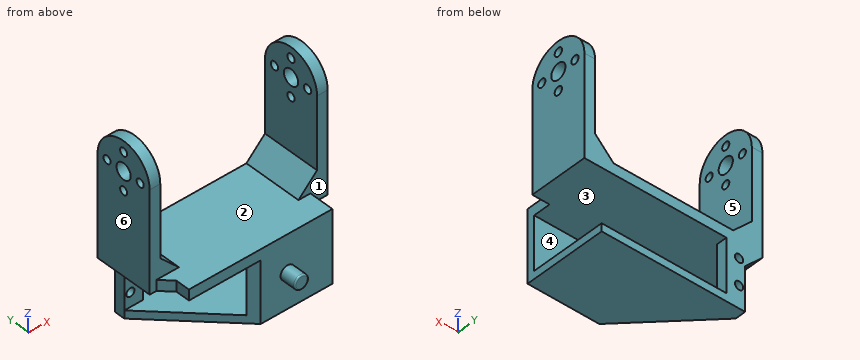
from build123d import *

# Parameters (mm, degrees)
BOSS_EXTRUDE1_DEPTH      = 22
SKETCH3_R                = 1.55
CUT_EXTRUDE1_DEPTH       = 30
CUT_EXTRUDE5_DEPTH       = 9
SKETCH11_R               = 1.55
CUT_EXTRUDE10_DEPTH      = 13
CUT_EXTRUDE11_START      = -10
CUT_EXTRUDE11_DEPTH      = 10
SKETCH13_R               = 3
SKETCH13_R_2             = 1.5
CUT_EXTRUDE12_DEPTH      = 85
FILLET1_SIZE             = 7
SKETCH14_W               = 54
SKETCH14_H               = 9.3
SKETCH14_W_2             = 7.05
SKETCH14_H_2             = 4
BOSS_EXTRUDE4_DEPTH      = 4
SKETCH17_W               = 7.05
SKETCH17_H               = 4
BOSS_EXTRUDE5_DEPTH      = 23.05
BOSS_EXTRUDE6_DEPTH      = 27.3
BOSS_EXTRUDE6_DEPTH_BACK = 4
SKETCH18_W               = 54
SKETCH18_H               = 2.95
SKETCH19_W               = 54
SKETCH19_H               = 2.8
BOSS_EXTRUDE7_DEPTH      = 21
FILLET2_SIZE             = 6.5
FILLET7_SIZE             = 4
SKETCH26_R               = 1.55
CUT_EXTRUDE18_DEPTH      = 11.5
CUT_EXTRUDE19_START      = -4
CUT_EXTRUDE19_OUTLINE_R  = 1.55
CUT_EXTRUDE19_DEPTH      = 4
CUT_EXTRUDE21_DEPTH      = 23.05
SKETCH31_R               = 2.625
BOSS_EXTRUDE8_DEPTH      = 6
FILLET8_R                = 0.5


# Read off the part's stored shape, not the designer's step: Cut-Extrude19
with BuildPart() as part:
    # Sketch1 → Boss-Extrude1 (new body)
    with BuildSketch(Plane(origin=(0, 0, 0), x_dir=(1, 0, 0), z_dir=(0, 1, 0))):
        Polygon((0, 0), (0, 50), (67, 50), (67, 0), (63, 0), (63, 46), (4, 46), (4, 0), align=None)
    extrude(amount=BOSS_EXTRUDE1_DEPTH)

    # Sketch3 → Cut-Extrude1 (cut)
    with BuildSketch(Plane(origin=(67, 0, 0), x_dir=(0, 0, -1), z_dir=(1, 0, 0))):
        with Locations((12.05, 11)):
            Circle(SKETCH3_R)
    extrude(amount=-CUT_EXTRUDE1_DEPTH, mode=Mode.SUBTRACT)

    # Sketch5 → Cut-Extrude5 (cut)
    with BuildSketch(Plane(origin=(67, 0, 0), x_dir=(0, 0, -1), z_dir=(1, 0, 0))):
        with BuildLine():
            Line((12.05, 22), (0, 22))
            Line((0, 22), (0, 0))
            Line((0, 0), (12.05, 0))
            ThreePointArc((12.05, 0), (1.05, 11), (12.05, 22))
        make_face()
    extrude(amount=-CUT_EXTRUDE5_DEPTH, mode=Mode.SUBTRACT)

    # Sketch11 → Cut-Extrude10 (cut)
    with BuildSketch(Plane(origin=(67, 0, 0), x_dir=(0, 0, -1), z_dir=(1, 0, 0))):
        with Locations((19.05, 11)):
            Circle(SKETCH11_R)
        with Locations((12.05, 18)):
            Circle(SKETCH11_R)
        with Locations((12.05, 4)):
            Circle(SKETCH11_R)
        with Locations((5.05, 11)):
            Circle(SKETCH11_R)
    extrude(amount=-CUT_EXTRUDE10_DEPTH, mode=Mode.SUBTRACT)

    # Sketch12 → Cut-Extrude11 (cut)
    with BuildSketch(Plane.ZY.offset(CUT_EXTRUDE11_START)):
        with BuildLine():
            Line((-12.05, 22), (0, 22))
            Line((0, 22), (0, 0))
            Line((0, 0), (-12.05, 0))
            ThreePointArc((-12.05, 0), (-1.05, 11), (-12.05, 22))
        make_face()
    extrude(amount=CUT_EXTRUDE11_DEPTH, mode=Mode.SUBTRACT)

    # Sketch13 → Cut-Extrude12 (cut)
    with BuildSketch(Plane.ZY):
        with Locations((-12.05, 11)):
            Circle(SKETCH13_R)
        with Locations((-19.05, 11)):
            Circle(SKETCH13_R_2)
        with Locations((-12.05, 4)):
            Circle(SKETCH13_R_2)
        with Locations((-5.05, 11)):
            Circle(SKETCH13_R_2)
        with Locations((-12.05, 18)):
            Circle(SKETCH13_R_2)
    extrude(amount=-CUT_EXTRUDE12_DEPTH, mode=Mode.SUBTRACT)

    # Fillet1
    fillet1_edges = [part.edges().sort_by_distance(p)[0] for p in [
        (63, 11, -46),
        (4, 11, -46),
    ]]
    chamfer(fillet1_edges, length=FILLET1_SIZE)

    # Sketch14 → Boss-Extrude4 (add)
    with BuildSketch(Plane(origin=(0, 0, -50), x_dir=(-1, 0, 0), z_dir=(0, 0, -1))):
        with Locations((-33.5, -4.65)):
            Rectangle(SKETCH14_W, SKETCH14_H)
        with Locations((-56.975, 20)):
            Rectangle(SKETCH14_W_2, SKETCH14_H_2)
        with Locations((-10.025, 20)):
            Rectangle(SKETCH14_W_2, SKETCH14_H_2)
    extrude(amount=-BOSS_EXTRUDE4_DEPTH)

    # Sketch17 → Boss-Extrude5 (add)
    with BuildSketch(Plane(origin=(0, 0, -50), x_dir=(-1, 0, 0), z_dir=(0, 0, -1))):
        with Locations((-56.975, 20)):
            Rectangle(SKETCH17_W, SKETCH17_H)
        with Locations((-10.025, 20)):
            Rectangle(SKETCH17_W, SKETCH17_H)
    extrude(amount=BOSS_EXTRUDE5_DEPTH)

    # Sketch18 → Boss-Extrude6 (add, two sides: drawn at the far end of the back side and taken through both)
    with BuildSketch(Plane.XZ.offset(-18).offset(-BOSS_EXTRUDE6_DEPTH_BACK)):
        with Locations((33.5, -71.575)):
            Rectangle(SKETCH18_W, SKETCH18_H)
    extrude(amount=BOSS_EXTRUDE6_DEPTH + BOSS_EXTRUDE6_DEPTH_BACK)

    # Sketch19 → Boss-Extrude7 (add)
    with BuildSketch(Plane(origin=(0, 0, -50), x_dir=(-1, 0, 0), z_dir=(0, 0, -1))):
        with Locations((-33.5, -7.9)):
            Rectangle(SKETCH19_W, SKETCH19_H)
    extrude(amount=BOSS_EXTRUDE7_DEPTH)

    # Fillet2
    fillet2_edges = [part.edges().sort_by_distance(p)[0] for p in [
        (60.5, 20, -50),
        (6.5, 20, -50),
    ]]
    chamfer(fillet2_edges, length=FILLET2_SIZE - 0.0001)  # a hair under: the kernel refuses the full size

    # Fillet7
    fillet7_edges = [part.edges().sort_by_distance(p)[0] for p in [
        (6.5, 0, -48),
    ]]
    chamfer(fillet7_edges, length=FILLET7_SIZE)

    # Sketch26 → Cut-Extrude18 (cut)
    with BuildSketch(Plane(origin=(0, 22, 0), x_dir=(1, 0, 0), z_dir=(0, 1, 0))):
        with Locations(Location((58.21, 64.77, 0), (0, 0, 270))):
            Circle(SKETCH26_R)
        with Locations(Location((58.21, 54.92, 0), (0, 0, 270))):
            Circle(SKETCH26_R)
        with Locations(Location((8.79, 54.92, 0), (0, 0, 270))):
            Circle(SKETCH26_R)
        with Locations(Location((8.79, 64.77, 0), (0, 0, 270))):
            Circle(SKETCH26_R)
    extrude(amount=-CUT_EXTRUDE18_DEPTH, mode=Mode.SUBTRACT)

    # Cut-Extrude19 outline → Cut-Extrude19 (cut)
    with BuildSketch(Plane(origin=(0, 22, 0), x_dir=(1, 0, 0), z_dir=(0, 1, 0)).offset(CUT_EXTRUDE19_START)):
        Polygon((53.45, 70.1), (53.45, 50), (67, 50), (60.5, 56.5), (60.5, 70.1), align=None)
        with Locations((58.21, 54.92)):
            Circle(CUT_EXTRUDE19_OUTLINE_R, mode=Mode.SUBTRACT)
        with Locations((58.21, 64.77)):
            Circle(CUT_EXTRUDE19_OUTLINE_R, mode=Mode.SUBTRACT)
    extrude(amount=CUT_EXTRUDE19_DEPTH, mode=Mode.SUBTRACT)

    # Sketch30 → Cut-Extrude21 (cut)
    with BuildSketch(Plane(origin=(0, 0, -73.05), x_dir=(-1, 0, 0), z_dir=(0, 0, -1))):
        Polygon((-6.5, 18), (-33.5, -9.3), (-6.5, -9.3), align=None)
    extrude(amount=-CUT_EXTRUDE21_DEPTH, mode=Mode.SUBTRACT)

    # Sketch31 → Boss-Extrude8 (add)
    with BuildSketch(Plane.XZ.offset(9.3)):
        with Locations(Location((43.6, -59.85, 0), (0, 0, 270))):
            Circle(SKETCH31_R)
    extrude(amount=BOSS_EXTRUDE8_DEPTH)

    # Fillet8
    fillet8_edges = [part.edges().sort_by_distance(p)[0] for p in [
        (43.6, -15.3, -57.225),
    ]]
    fillet(fillet8_edges, radius=FILLET8_R)


solid = part.part
Verification items for the finished model (mm, model axes). Face numbers are marked on the shaded views. A direction names the side the tool comes from. Coordinates: 2 decimals unless noted, no trailing zeros. Write each loop counter-clockwise with the first axis right and the second up, starting at its lowest first coordinate (ties: lowest second). Pieces come first, ordered by that corner, then holes. Notation, with made-up numbers: (22.5, -32) -> (71.5, -32) arc R32 cw to (71.5, -5) -> close; hole circle Ø6 at (85, 8.5). An arc over 180 degrees is marked (long way). One line per item, written item: value. Start each with the question number.
Q1. Go/stop test with flat-tipped pins: P1, Ø14, axis at x = 36, y = 9.5, coming from the +Z side; P2, Ø12, axis at x = 62.5, z = -31, coming from the -Y side; P3, Ø6, axis at x = 49, z = -59.5, coming from the +Y side. Record where each tip stops, or that it passes through.
Q2. Mould release check, pull along Z, two halves, no side actions. Record for the marked faces 1, 2 and 3: pulls with the +Z half, pulls with the -Z half, needs draft (parallel to the pull), parting line crosses it, or undercut.
Q3. Thickness scan on L1, parallel to Y at x = 64.05, z = -12.05; L2, parallel to X at y = 16.5, z = -10.5; L3, parallel to Z at x = 20.5, y = 8. Record the ranges inside material, lowest first. Write a range as from..to.
Q4. Access from +Z, -Z, +X, -X, +Y, -Y to the whole of each face (thin tool, end or side, straight path). Record for the marked faces 4, 5 and 6.
Q5. Cross-section at C-C on x = 38. Enter the section's corners in (y, z).
Q6. Cross-section at A-A on z = -59.85. Enter the section's corners in (x, y) (3 decimals).
Q7. Cross-section at D-D on y = 4. Enter the section's corners in (x, z).
Q8. Cross-section at B-B on x = 26. Enter the section's corners in (y, z).
Checked values:
1. P1: stops at z = -46
1. P2: stops at y = 0
1. P3: stops at y = -6.5
2. face 1: needs draft
2. face 2: pulls with the +Z half
2. face 3: undercut
3. L1: y = 0..2.45, 5.55..8, 14..16.45, 19.55..22
3. L2: x = 0..4, 63..67
3. L3: z = -73.05..-70.1, -50..-46
4. face 4: +X, -X, +Y
4. face 5: +Z, +Y, -Y
4. face 6: +Z, -Z, -X, +Y, -Y
5. outline: (-9.3, -73.05) -> (22, -73.05) -> (22, -70.1) -> (-6.5, -70.1) -> (-6.5, -50) -> (22, -50) -> (22, -46) -> (-9.3, -46) -> close
6. outline: (6.5, 18) -> (13.55, 18) -> (13.55, 22) -> (6.5, 22) -> close; (30.731, -6.5) -> (33.5, -9.3) -> (40.975, -9.3) -> (40.975, -14.8) arc R0.5 ccw to (41.475, -15.3) -> (45.725, -15.3) arc R0.5 ccw to (46.225, -14.8) -> (46.225, -9.3) -> (60.5, -9.3) -> (60.5, -6.5) -> close
7. outline: (0, -50) -> (67, -50) -> (67, -13.6) -> (63, -13.6) -> (63, -39) -> (56, -46) -> (11, -46) -> (4, -39) -> (4, -13.55) -> (0, -13.55) -> close; (0, -10.55) -> (4, -10.55) -> (4, -3.56) -> (0, -3.56) -> close; (20.35, -73.05) -> (60.5, -73.05) -> (60.5, -70.1) -> (20.35, -70.1) -> close; (63, -10.5) -> (67, -10.5) -> (67, -3.56) -> (63, -3.56) -> close
8. outline: (-9.3, -50) -> (22, -50) -> (22, -46) -> (-9.3, -46) -> close; (-1.72, -73.05) -> (22, -73.05) -> (22, -70.1) -> (-1.72, -70.1) -> close
